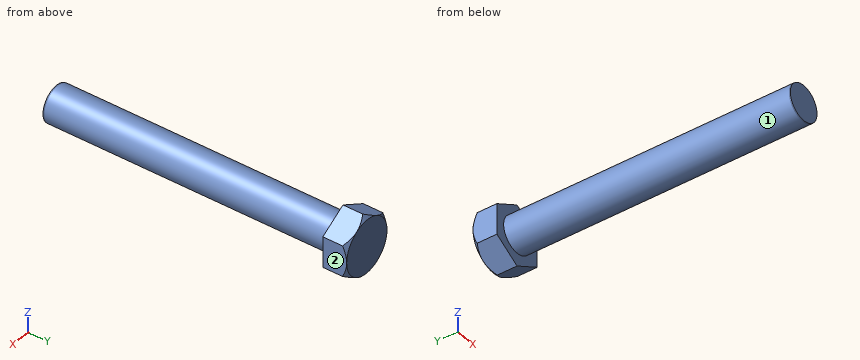
```python
from build123d import *

# Parameters (mm, degrees)
BOSS_EXTRUDE1_DEPTH = 6.35
SKETCH2_R           = 4.7625
BOSS_EXTRUDE2_DEPTH = 76.2
SKETCH3_OUTSIDE_W   = 74.018
SKETCH3_OUTSIDE_H   = 76.23
SKETCH3_OUTSIDE_R   = 7.1501
CUT_EXTRUDE1_DEPTH  = 20.32
CUT_EXTRUDE1_TAPER  = 45
CHAMFER1_SIZE       = 0.254
CHAMFER1_SIZE2      = 0.022222121


with BuildPart() as part:
    # Sketch1 → Boss-Extrude1 (new body)
    with BuildSketch(Plane(origin=(0, 0, 0), x_dir=(1, 0, 0), z_dir=(0, 1, 0))):
        Polygon((0, 8.256224319), (-7.1501, 4.12811216), (-7.1501, -4.12811216), (0, -8.256224319), (7.1501, -4.12811216), (7.1501, 4.12811216), align=None)
    extrude(amount=BOSS_EXTRUDE1_DEPTH)

    # Sketch2 → Boss-Extrude2 (add)
    with BuildSketch(Plane.XZ):
        Circle(SKETCH2_R)
    extrude(amount=BOSS_EXTRUDE2_DEPTH)

    # Sketch3 outside → Cut-Extrude1 (cut)
    with BuildSketch(Plane(origin=(0, 6.35, 0), x_dir=(1, 0, 0), z_dir=(0, 1, 0))):
        Rectangle(SKETCH3_OUTSIDE_W, SKETCH3_OUTSIDE_H)
        Circle(SKETCH3_OUTSIDE_R, mode=Mode.SUBTRACT)
    extrude(amount=-CUT_EXTRUDE1_DEPTH, taper=CUT_EXTRUDE1_TAPER, mode=Mode.SUBTRACT)

    # Chamfer1
    chamfer1_edges = [part.edges().sort_by_distance(p)[0] for p in [
        (-4.7625, -76.2, 0),
    ]]
    chamfer1_side = [part.faces().sort_by_distance(p)[0] for p in [
        (-4.7625, -38.1, 0),
    ]]
    chamfer(chamfer1_edges, length=CHAMFER1_SIZE, length2=CHAMFER1_SIZE2, reference=chamfer1_side[0])


solid = part.part
```
Verification items for the finished model (mm, model axes). Face numbers are marked on the shaded views. A direction names the side the tool comes from. Coordinates: 2 decimals unless noted, no trailing zeros. Loops run counter-clockwise (first coordinate to the right, second up) from the corner with the lowest first, then second, coordinate; pieces in that order, holes last. Notation, with made-up numbers: (53.25, 27.5) -> (104.25, 27.5) arc R7 ccw to (104.25, 40.5) -> close; hole circle Ø3 at (-16, 51.25). An arc over 180 degrees is marked (long way). Answer in a Markdown table with one row per item.
1) Depth check by flat-ended pin: P1, Ø2, axis at x = -3, y = -63, coming from the +Z side; P2, Ø3, axis at y = -46.5, z = -5.5, coming from the +X side; P3, Ø6, axis at x = -3, y = -40, coming from the +Z side. Enter the tip coordinate at first touch or a pass-through.
The answers:
| item | result |
|---|---|
| P1 | stops at z = 4.32 |
| P2 | stops at x = 2.58 |
| P3 | stops at z = 4.76 |
2) Access from +Z, -Z, +X, -X, +Y, -Y to the whole of each face (thin tool, end or side, straight path). Record for the marked faces 1 and 2.
The answers:
| item | result |
|---|---|
| face 1 | -Y |
| face 2 | +Z, -Z, +X, +Y, -Y |
3) Scan lines: line 1 along Z through (x, y) = (0, -43.5); line 2 along Y through (x, z) = (-1, -5.5); line 3 along X through (y, z) = (-34.5, -0.5). Record each from-to range of solid material in increasing order. Write a range as from..to.
The answers:
| item | result |
|---|---|
| line 1 | z = -4.76..4.76 |
| line 2 | y = 0..6.35 |
| line 3 | x = -4.74..4.74 |
4) Section check A-A (y = -63). Record the cut outline in (x, z) (1 decimal).
The answers:
| item | result |
|---|---|
| outline | circle Ø9.5 at (0, 0) |
